```python
from build123d import *

# Parameters (mm, degrees)
SKETCH1_R           = 1.6
BOSS_EXTRUDE1_DEPTH = 17
SKETCH2_R           = 2.1
CUT_EXTRUDE1_DEPTH  = 27.305892876


with BuildPart() as part:
    # Sketch1 → Boss-Extrude1 (new body)
    with BuildSketch(Plane.XY.offset(5)):
        with BuildLine():
            Line((-8, -4), (0, -4))
            ThreePointArc((0, -4), (4, 0), (0, 4))
            Line((0, 4), (-8, 4))
            ThreePointArc((-8, 4), (-12, 0), (-8, -4))
        make_face()
        Circle(SKETCH1_R, mode=Mode.SUBTRACT)
    extrude(amount=BOSS_EXTRUDE1_DEPTH)

    # Sketch2 → Cut-Extrude1 (cut, through all)
    with BuildSketch(Plane(origin=(0, 4, 0), x_dir=(1, 0, 0), z_dir=(0, 1, 0))):
        with Locations(Location((-6, -13.5, 0), (0, 0, 197.752790162))):
            Circle(SKETCH2_R)
    extrude(amount=-CUT_EXTRUDE1_DEPTH, mode=Mode.SUBTRACT)


solid = part.part
```
Work out the finished part from the listing and answer in its coordinate system (mm). Round coordinates to 2 decimals unless told otherwise and drop trailing zeros. Write each loop counter-clockwise with the first axis right and the second up, starting at its lowest first coordinate (ties: lowest second). Pieces come first, ordered by that corner, then holes. Notation, with made-up numbers: (79.25, -1.5) - (108.25, -1.5) arc R18 ccw to (108.25, 11.5) - close; hole circle Ø4 at (-5.75, 10.5). An arc over 180 degrees is marked (long way). Return JSON: item names as keys, results as strings. Group by question number.
Q1. Find the intervals of material crossed by L1, parallel to Z at x = -6, y = -2; L2, parallel to X at y = -0.25, z = 13.5; L3, parallel to X at y = -2, z = 13.5, in increasing order.
Q2. The part is cut by section B-B on y = 0. Write down the section's boundary in (x, z), then the cut area to 3 significant figures.
Q3. The part is cut by section C-C on x = -6. Write down the section's boundary in (y, z).
Q4. The mould has two halves that part along X. Classify faces 1 (the cylindrical face through (4, 0, 13)), 2 (the cylindrical face through (-12, 0, 13)), 3 (the cylindrical face through (-6.54, 0.06, 15.53)), 4 (the flat face through (-4, 0, 5)): released by +X, released by -X, zero draft, split by the parting line, or undercut.
Q5. The part is cut by section A-A on z = 13.25. Write down the section's boundary in (x, y).
Q6. Each of these flat-tipped pins is pushed along its axis until it touches: pin 1 Ø2 at (y, z) = (2, 14.5) entering from +X; pin 2 Ø4 at (y, z) = (2.5, 13) entering from -X. Where does it stop, or does it pass through?
Q7. The part is cut by section D-D on z = 20.5. Write down the section's boundary in (x, y), then the cut area to 3 significant figures.
Solved:
{
 "1": {"L1": "5 to 11.4, 15.6 to 22", "L2": "-11.99 to -8.1, -3.9 to -1.58, 1.58 to 3.99", "L3": "-11.46 to -8.1, -3.9 to 3.46"},
 "2": {"outline": "(-12, 5) - (-1.6, 5) - (-1.6, 22) - (-12, 22) - close; (1.6, 5) - (4, 5) - (4, 22) - (1.6, 22) - close; hole circle Ø4.2 at (-6, 13.5)", "area": "204 mm²"},
 "3": {"outline": "(-4, 5) - (4, 5) - (4, 11.4) - (-4, 11.4) - close; (-4, 15.6) - (4, 15.6) - (4, 22) - (-4, 22) - close"},
 "4": {"face 1": "released by +X", "face 2": "released by -X", "face 3": "undercut", "face 4": "zero draft"},
 "5": {"outline": "(-8.09, -4) - (-8.09, 4) arc R4 ccw to start; (-3.91, -4) - (0, -4) arc R4 ccw to (0, 4) - (-3.91, 4) - close; hole circle Ø3.2 at (0, 0)"},
 "6": {"pin 1": "x = 3.87", "pin 2": "x = -11.97"},
 "7": {"outline": "(-8, -4) - (0, -4) arc R4 ccw to (0, 4) - (-8, 4) arc R4 ccw to start; hole circle Ø3.2 at (0, 0)", "area": "106 mm²"}
}
